Geometry: final body of the model. Coordinates: model frame, mm. A direction names the side the tool comes from. Coordinates: 2 decimals unless noted, no trailing zeros. Order: outer loops, then holes, each group sorted by start corner. A loop starts at its lowest first (then second) coordinate and runs counter-clockwise, first axis right, second up. Notation, with made-up numbers: (39.5, 4.5) -> (80.5, 4.5) arc R35 cw to (80.5, 42.5) -> close; hole circle Ø1 at (-24, -15.5). An arc over 180 degrees is marked (long way). Use CSV: the item, a comma, the result in double quotes. Start each with the question number.
from build123d import *

# Parameters (mm, degrees)
F0_R     = 39
F0_R_2   = 30
F1_DEPTH = 5
F2_R     = 38
F2_R_2   = 31
F3_DEPTH = 0.5


# Not quite as in the source:
# - a pattern or mirror of a feature is missing from the dataset's text; its kind, count and spacing are read off the source's solid


with BuildPart() as f1:
    # F0 (on Top) → F1 (new body, symmetric)
    with BuildSketch(Plane.XY):
        Circle(F0_R)
        Circle(F0_R_2, mode=Mode.SUBTRACT)
    extrude(amount=F1_DEPTH, both=True)

    # F2 (on face) → F3 (cut)
    with BuildSketch(Plane.XY.offset(5)):
        Circle(F2_R)
        Circle(F2_R_2, mode=Mode.SUBTRACT)
    f3 = extrude(amount=-F3_DEPTH, mode=Mode.SUBTRACT)

    # F3_copies: F3 across plane
    add(f3.mirror(Plane(origin=(0, 0, 0), x_dir=(-1, 0, 0), z_dir=(0, 0, -1))), mode=Mode.SUBTRACT)


solid = f1.part
(1) Line query: line 1 (Y direction, x = 0, z = 4.8); line 2 (Y direction, x = 0, z = 0.5); line 3 (Z direction, x = 33, y = -4.5). Output: solid intervals per line, ascending. Write a range as from..to.
(2) Section A-A (y = 0). Return loops of the section in (x, z), then the cut area to 3 significant figures.
(3) Section D-D (x = -33). Return loops of the section in (y, z).
(4) Section C-C (z = 0). Return loops of the section in (x, y).
(5) Access query for faces 5 (the face through (-14, -28, 4.5)), 6 (the face through (-14, -28, -4.5)), 7 (the face through (-12, 28, 5)). Directions: +Z, -Z, +X, -X, +Y, -Y. A direction counts if a zero-diameter tool reaches every point of the face in a straight line with its end or side. Return the directions, or none.
(6) First-contact query: pin 1 (6 mm diameter, centred on x = -16, z = -3.5, fed in from -Y); pin 2 (2 mm diameter, centred on y = 3, z = 1, fed in from -X); pin 3 (5 mm diameter, centred on x = -7.5, z = 0, fed in from -Y); pin 4 (10 mm diameter, centred on x = -11, y = -29.5, fed in from +Z). Flat tips, straight axial feed; report the tip coordinate or a pass-through.
(7) Mould query, pull axis Y, two halves, no side actions, for faces 1 (the face through (-5.077, 38.668, 0.07)), 2 (the face through (-12, 28, -5)), 3 (the face through (17.535, -33.713, 4.754)), 4 (the face through (-4.036, 30.736, 4.754)). Classes: pulls with the +Y half, pulls with the -Y half, needs draft (parallel to the pull), parting line crosses it, or undercut.
Check sheet entries:
1,line 1,"y = -39..-38, -31..-30, 30..31, 38..39"
1,line 2,"y = -39..-30, 30..39"
1,line 3,"z = -4.5..4.5"
2,outline,"(-39, -5) -> (-38, -5) -> (-38, -4.5) -> (-31, -4.5) -> (-31, -5) -> (-30, -5) -> (-30, 5) -> (-31, 5) -> (-31, 4.5) -> (-38, 4.5) -> (-38, 5) -> (-39, 5) -> close; (30, -5) -> (31, -5) -> (31, -4.5) -> (38, -4.5) -> (38, -5) -> (39, -5) -> (39, 5) -> (38, 5) -> (38, 4.5) -> (31, 4.5) -> (31, 5) -> (30, 5) -> close"
2,area,"166 mm^2"
3,outline,"(-20.78, -5) -> (-18.84, -5) -> (-18.84, -4.5) -> (18.84, -4.5) -> (18.84, -5) -> (20.78, -5) -> (20.78, 5) -> (18.84, 5) -> (18.84, 4.5) -> (-18.84, 4.5) -> (-18.84, 5) -> (-20.78, 5) -> close"
4,outline,"circle Ø78 at (0, 0); hole circle Ø60 at (0, 0)"
5,face 5,"+Z"
5,face 6,"-Z"
5,face 7,"+Z, +X, -X, +Y, -Y"
6,pin 1,"stops at y = -36.77"
6,pin 2,"stops at x = -38.95"
6,pin 3,"stops at y = -38.68"
6,pin 4,"stops at z = 5"
7,face 1,"parting line crosses it"
7,face 2,"needs draft"
7,face 3,"undercut"
7,face 4,"undercut"
